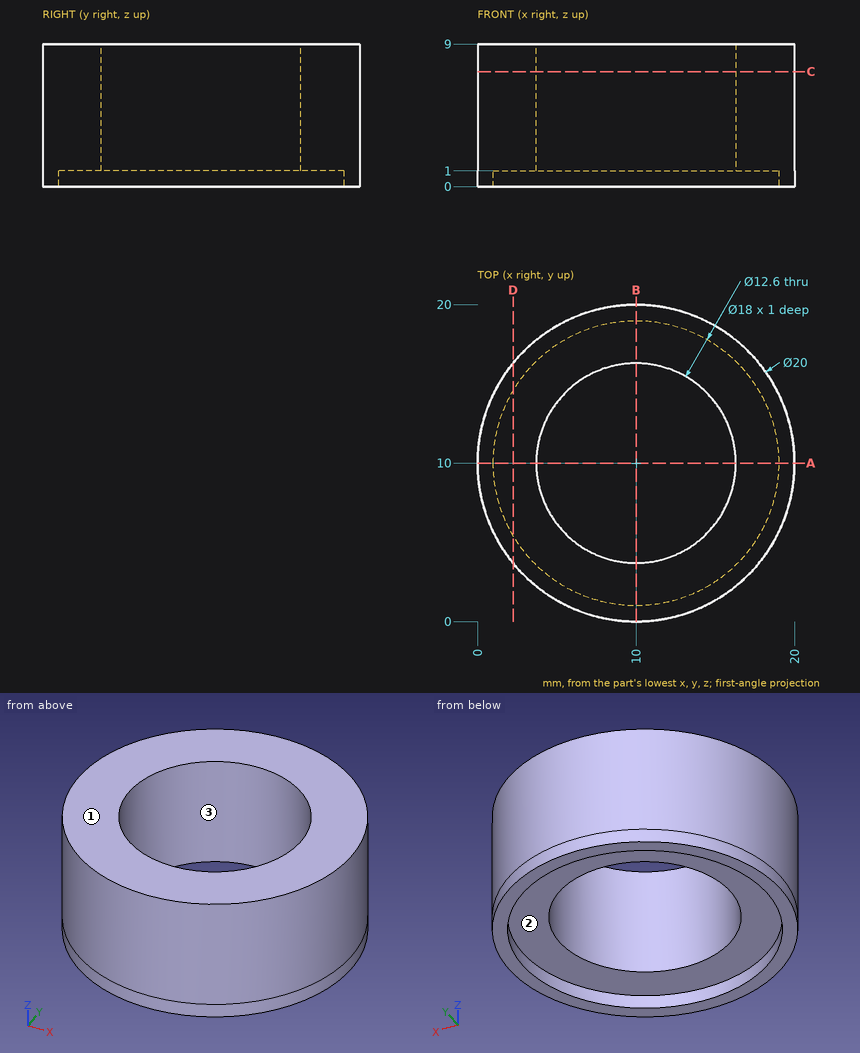
Verification items for this drawing (mm, ordinates from the low corner). Round coordinates to 2 decimals unless told otherwise and drop trailing zeros. Order: outer loops, then holes, each group sorted by start corner. A loop starts at its lowest first (then second) coordinate and runs counter-clockwise, first axis right, second up.
1) Depth check by flat-ended pin: pin 1 (1.5 mm diameter, centred on x = 17, z = 1.5, fed in from +Y); pin 2 (10 mm diameter, centred on x = 10, y = 10, fed in from -Z); pin 3 (1 mm diameter, centred on x = 15, z = 4, fed in from -Y). Enter the tip coordinate at first touch or a pass-through.
Geometry says:
pin 1: stops at y = 17.81
pin 2: passes through
pin 3: stops at y = 1.07
2) Draft check along X on the marked faces 1, 2 and 3. Enter one of: +X half, -X half, draft (parallel to the pull), parting line (faces both ways), or undercut.
Geometry says:
face 1: draft
face 2: undercut
face 3: undercut
3) Cross-section at A-A, the plane y = 10. Record the cut outline in (x, z).
Geometry says:
outline: (0, 0) - (1, 0) - (1, 1) - (3.7, 1) - (3.7, 9) - (0, 9) - close; (16.3, 1) - (19, 1) - (19, 0) - (20, 0) - (20, 9) - (16.3, 9) - close
4) Material ranges on line 1 (Y direction, x = 10, z = 0.35); line 2 (Y direction, x = 10, z = 4); line 3 (Z direction, x = 16.25, y = 12), recorded low to high.
Geometry says:
line 1: y = 0 to 1, 19 to 20
line 2: y = 0 to 3.7, 16.3 to 20
line 3: z = 1 to 9
5) Cross-section at D-D, the plane x = 2.25. Record the cut outline in (y, z).
Geometry says:
outline: (3.68, 0) - (5.42, 0) - (5.42, 1) - (14.58, 1) - (14.58, 0) - (16.32, 0) - (16.32, 9) - (3.68, 9) - close
6) Cross-section at C-C, the plane z = 7.25. Record the cut outline in (x, y).
Geometry says:
outline: circle Ø20 at (10, 10); hole circle Ø12.6 at (10, 10)
